Autodesk Fusion 360 part; units mm, degrees
sketch "Sketch1" plane through (0, 0, 0) normal (0, 1, 0) x (1, 0, 0)
  line L0 (57.15, -34.925) -> (-57.15, -34.925)
  line L1 (-57.15, -34.925) -> (-57.15, 34.925)
  line L2 (-57.15, 34.925) -> (57.15, 34.925)
  line L3 (57.15, 34.925) -> (57.15, -34.925)
  line L4 (57.15, -34.925) -> (-57.15, 34.925) construction
  line L5 (-57.15, -34.925) -> (57.15, 34.925) construction
  dimension "d1" = 114.3
  dimension "d2" = 69.85
extrude "Extrude1" add sketch "Sketch1" along normal blind 44.45
sketch "Sketch10" plane through (0, 44.45, 0) normal (0, 1, 0) x (-1, 0, 0)
  line L0 (-57.15, -34.925) -> (57.15, -34.925)
  line L1 (57.15, -34.925) -> (57.15, 34.925)
  line L2 (57.15, 34.925) -> (-57.15, 34.925)
  line L3 (-57.15, 34.925) -> (-57.15, -34.925)
  line L4 (-73.025, 44.45) -> (73.025, 44.45)
  line L5 (73.025, 44.45) -> (73.025, -44.45)
  line L6 (73.025, -44.45) -> (-73.025, -44.45)
  line L7 (-73.025, -44.45) -> (-73.025, 44.45)
  line L8 (-73.025, 44.45) -> (73.025, -44.45) construction
  line L9 (73.025, 44.45) -> (-73.025, -44.45) construction
  dimension "d55" = 146.05
  dimension "d56" = 88.9
extrude "Extrude14" add sketch "Sketch10" along normal blind 5.08 contours L0 L1 L2 L3 | L4 L5 L6 L7
sketch "Sketch11" plane through (0, 49.53, 0) normal (0, 1, 0) x (-1, 0, 0)
  line L0 (-73.025, -44.45) -> (73.025, -44.45)
  line L1 (73.025, -44.45) -> (73.025, 44.45)
  line L2 (73.025, 44.45) -> (-73.025, 44.45)
  line L3 (-73.025, 44.45) -> (-73.025, -44.45)
  line L4 (57.15, -34.925) -> (-57.15, -34.925)
  line L5 (-57.15, -34.925) -> (-57.15, 34.925)
  line L6 (-57.15, 34.925) -> (57.15, 34.925)
  line L7 (57.15, 34.925) -> (57.15, -34.925)
  line L8 (63.5, -38.1) -> (-63.5, -38.1)
  line L9 (-63.5, -38.1) -> (-63.5, 38.1)
  line L10 (-63.5, 38.1) -> (63.5, 38.1)
  line L11 (63.5, 38.1) -> (63.5, -38.1)
  line L12 (63.5, -38.1) -> (-63.5, 38.1) construction
  line L13 (-63.5, -38.1) -> (63.5, 38.1) construction
  dimension "d61" = 127
  dimension "d62" = 76.2
sketch "Sketch27" plane through (0, 49.53, 0) normal (0, 1, 0) x (-1, 0, 0)
  line L0 (-73.025, -44.45) -> (73.025, -44.45)
  line L1 (73.025, -44.45) -> (73.025, 44.45)
  line L2 (73.025, 44.45) -> (-73.025, 44.45)
  line L3 (-73.025, 44.45) -> (-73.025, -44.45)
  line L4 (57.15, -34.925) -> (-57.15, -34.925)
  line L5 (-57.15, -34.925) -> (-57.15, 34.925)
  line L6 (-57.15, 34.925) -> (57.15, 34.925)
  line L7 (57.15, 34.925) -> (57.15, -34.925)
  line L8 (-54.61, 32.385) -> (54.61, 32.385)
  line L9 (54.61, 32.385) -> (54.61, -32.385)
  line L10 (54.61, -32.385) -> (-54.61, -32.385)
  line L11 (-54.61, -32.385) -> (-54.61, 32.385)
  dimension "d89" = 2.54
extrude "Extrude22" cut sketch "Sketch27" against normal blind 48.26 contours L8 L9 L10 L11
sketch "Sketch28" plane through (0, 49.53, 0) normal (0, 1, 0) x (-1, 0, 0)
  line L0 (54.61, 32.385) -> (54.61, -32.385)
  line L1 (54.61, -32.385) -> (-54.61, -32.385)
  line L2 (-54.61, -32.385) -> (-54.61, 32.385)
  line L3 (-54.61, 32.385) -> (54.61, 32.385)
  line L4 (-73.025, -44.45) -> (73.025, -44.45)
  line L5 (73.025, -44.45) -> (73.025, 44.45)
  line L6 (73.025, 44.45) -> (-73.025, 44.45)
  line L7 (-73.025, 44.45) -> (-73.025, -44.45)
  circle A0 centre (63.373, 0) radius 1.905
  line L8 (0, 0) -> (0, 7.62)
  circle A1 centre (-63.373, 0) radius 1.905
  dimension "d92" = 3.81
  dimension "d93" = 9.652
extrude "Extrude23" cut sketch "Sketch28" against normal blind 38.1 contours A0 | A1
sketch "Sketch29" plane through (0, 0, 34.925) normal (0, 0, 1) x (1, 0, 0)
  line L0 (-57.15, 0) -> (57.15, 0)
  line L1 (57.15, 0) -> (57.15, 44.45)
  line L2 (57.15, 44.45) -> (-57.15, 44.45)
  line L3 (-57.15, 44.45) -> (-57.15, 0)
  line L4 (-22.698, 21.1911) -> (-12.538, 21.1911)
  line L5 (-12.538, 21.1911) -> (-12.538, 13.5711)
  line L6 (-12.538, 13.5711) -> (-22.698, 13.5711)
  line L7 (-22.698, 13.5711) -> (-22.698, 21.1911)
  circle A0 centre (15.9589, 19.9606) radius 5.715
  dimension "d96" = 10.16
  dimension "d97" = 7.62
  dimension "d98" = 11.43
sketch "Sketch30" plane through (0, 0, -34.925) normal (0, 0, -1) x (-1, 0, 0)
  line L0 (-57.15, 0) -> (57.15, 0)
  line L1 (57.15, 0) -> (57.15, 44.45)
  line L2 (57.15, 44.45) -> (-57.15, 44.45)
  line L3 (-57.15, 44.45) -> (-57.15, 0)
  line L4 (40.0812, 6.9441) -> (27.3812, 6.9441)
  line L5 (27.3812, 6.9441) -> (27.3812, 17.1041)
  line L6 (27.3812, 17.1041) -> (40.0812, 17.1041)
  line L7 (40.0812, 17.1041) -> (40.0812, 6.9441)
  dimension "d114" = 12.7
  dimension "d115" = 10.16
sketch "Sketch31" plane through (57.15, 0, 0) normal (1, 0, 0) x (0, 0, -1)
  line L0 (-34.925, 0) -> (34.925, 0)
  line L1 (34.925, 0) -> (34.925, 44.45)
  line L2 (34.925, 44.45) -> (-34.925, 44.45)
  line L3 (-34.925, 44.45) -> (-34.925, 0)
  line L4 (6.35, 12.7) -> (-6.35, 12.7)
  line L5 (-6.35, 12.7) -> (-6.35, 17.78)
  line L6 (-6.35, 17.78) -> (6.35, 17.78)
  line L7 (6.35, 17.78) -> (6.35, 12.7)
  line L8 (6.35, 12.7) -> (-6.35, 17.78) construction
  line L9 (-6.35, 12.7) -> (6.35, 17.78) construction
  point P0 (0, 15.24)
  dimension "d101" = 12.7
  dimension "d102" = 5.08
extrude "Extrude24" cut sketch "Sketch29" against normal blind 40.64 contours L4 L5 L6 L7 | A0
extrude "Extrude25" cut sketch "Sketch30" against normal blind 33.02 contours L4 L5 L6 L7
extrude "Extrude26" cut sketch "Sketch31" against normal blind 33.02 contours L4 L5 L6 L7
sketch "Sketch32" plane through (0, 1.27, 0) normal (0, 1, 0) x (-1, 0, 0)
  line L0 (-54.61, -32.385) -> (54.61, -32.385)
  line L1 (54.61, -32.385) -> (54.61, 32.385)
  line L2 (54.61, 32.385) -> (-54.61, 32.385)
  line L3 (-54.61, 32.385) -> (-54.61, -32.385)
  circle A0 centre (43.18, -5.08) radius 1.1938
  line L4 (43.18, -5.08) -> (-30.0482, -5.08)
  circle A1 centre (-30.0482, -5.08) radius 1.1938
  dimension "d109" = 2.3876
  dimension "d110" = 73.2282
  dimension "d111" = 2.3876
extrude "Extrude27" cut sketch "Sketch32" against normal blind 10.16 contours A0 | A1
Geometry: final body of the model. Coordinates: model frame, mm. A direction names the side the tool comes from. Give positions to 0.01 mm unless a question says otherwise; leave off trailing zeros. Loops run counter-clockwise (first coordinate to the right, second up) from the corner with the lowest first, then second, coordinate; pieces in that order, holes last. Notation, with made-up numbers: M 33,59.5 L 75,59.5 A28 ccw 75,97.5 Z; hole C 75.25,34 d1. An arc over 180 degrees is marked long. Put each result on its own line as item: value. Start each with the question number.
1) Cut plane C-C (z = -15). Output: boundary loops of the cut face in (x, y) (3 decimals), then the cut area to 3 significant figures.
2) Contact query for flat-ended pins moving along their axis: pin 1 (3 mm diameter, centred on y = 17, z = 33, fed in from -X); pin 2 (1.5 mm diameter, centred on x = 29, y = 39.5, fed in from -Z) (3 decimals); pin 3 (2.5 mm diameter, centred on x = -43.18, z = -5.08, fed in from +Y); pin 4 (5 mm diameter, centred on x = -1.5, z = -30.5, fed in from +Y). Output: stop coordinate, or through.
3) Ray query, line 1 along Z through (x, y) = (-43.18, 0.75) (3 decimals); line 2 along Z through (x, y) = (37.5, 14) (3 decimals); line 3 along X through (y, z) = (4, 3). Return the intervals inside material, ascending.
4) Cut plane A-A (z = 0). Output: boundary loops of the cut face in (x, y) (3 decimals), then the cut area to 3 significant figures.
5) Access query for faces 1 (the flat face through (1, 44.45, -39)), 2 (the flat face through (1, 26, 32.385)), 3 (the flat face through (-57.15, 22, 0)), 4 (the flat face through (-1, 22, -34.925)). Directions: +Z, -Z, +X, -X, +Y, -Y. A direction counts if a zero-diameter tool reaches every point of the face in a straight line with its end or side. Return the directions, or none.
6) Cut plane B-B (x = -7.5). Output: boundary loops of the cut face in (y, z) (3 decimals).
7) Pull-direction query (Z, two-part tool) for faces 5 (the flat face through (-1, 26, -32.385)), 6 (the flat face through (1, 22, 34.925)), 7 (the cylindrical face through (21.41, 21.68, 33.67)); classes: pulls with the +Z half, pulls with the -Z half, needs draft (parallel to the pull), parting line crosses it, or undercut.
Verdict:
1. outline: M -73.025,44.45 L -57.15,44.45 L -57.15,0 L 57.15,0 L 57.15,44.45 L 73.025,44.45 L 73.025,49.53 L 54.61,49.53 L 54.61,1.27 L -54.61,1.27 L -54.61,49.53 L -73.025,49.53 Z
1. area: 552 mm2
2. pin 1: x = -57.15
2. pin 2: z = -34.925
2. pin 3: y = 1.27
2. pin 4: y = 49.53
3. line 1: -34.925 to -6.274, -3.886 to 34.925
3. line 2: -34.925 to -32.385, 32.385 to 34.925
3. line 3: -57.15 to -54.61, 54.61 to 57.15
4. outline: M -73.025,44.45 L -65.278,44.45 L -65.278,49.53 L -73.025,49.53 Z; M -61.468,44.45 L -57.15,44.45 L -57.15,0 L 57.15,0 L 57.15,12.7 L 54.61,12.7 L 54.61,1.27 L -54.61,1.27 L -54.61,49.53 L -61.468,49.53 Z; M 54.61,17.78 L 57.15,17.78 L 57.15,44.45 L 61.468,44.45 L 61.468,49.53 L 54.61,49.53 Z; M 65.278,44.45 L 73.025,44.45 L 73.025,49.53 L 65.278,49.53 Z
4. area: 500 mm2
5. face 1: -Y
5. face 2: +Y
5. face 3: +Z, -Z, -X, -Y
5. face 4: -Z, +X, -X, -Y
6. outline: M 0,-34.925 L 44.45,-34.925 L 44.45,-44.45 L 49.53,-44.45 L 49.53,-32.385 L 1.27,-32.385 L 1.27,32.385 L 49.53,32.385 L 49.53,44.45 L 44.45,44.45 L 44.45,34.925 L 0,34.925 Z
7. face 5: undercut
7. face 6: pulls with the +Z half
7. face 7: needs draft
